Autodesk Inventor part; units mm, degrees
ref_plane "YZ Plane" through (0, 0, 0) normal (1, 0, 0) x (0, 1, 0)
ref_plane "XZ Plane" through (0, 0, 0) normal (0, 1, 0) x (-1, 0, 0)
ref_plane "XY Plane" through (0, 0, 0) normal (0, 0, 1) x (1, 0, 0)
sketch "Sketch1" plane through (0, 0, 0) normal (0, 1, 0) x (-1, 0, 0)
  line L0 (0, 0) -> (-75, 0)
  line L1 (-75, 0) -> (-75, -250)
  line L2 (-75, -250) -> (0, -250)
  line L3 (0, -250) -> (0, 0)
  line L4 (-20, -10) -> (-60, -10)
  line L5 (-60, -10) -> (-60, -15)
  line L6 (-60, -15) -> (-20, -15)
  line L7 (-20, -15) -> (-20, -10)
  line L8 (-75, -125) -> (0, -125) construction
  line L9 (-20, -240) -> (-60, -240)
  line L10 (-60, -240) -> (-60, -235)
  line L11 (-60, -235) -> (-20, -235)
  line L12 (-20, -235) -> (-20, -240)
  line L13 (-75, -35) -> (-265, -35)
  line L14 (-265, -35) -> (-265, -215)
  line L15 (-265, -215) -> (-75, -215)
  line L16 (-75, -215) -> (-75, -35)
  line L17 (-265, -65) -> (-270, -65)
  line L18 (-270, -65) -> (-270, -185)
  line L19 (-270, -185) -> (-265, -185)
  line L20 (-265, -185) -> (-265, -65)
  line L21 (0, -75) -> (-5, -75)
  line L22 (-5, -75) -> (-5, -175)
  line L23 (-5, -175) -> (0, -175)
  line L24 (0, -175) -> (0, -75)
  line L25 (-125, -35) -> (-210, -35)
  line L26 (-210, -35) -> (-210, -15)
  line L27 (-210, -15) -> (-125, -15)
  line L28 (-125, -15) -> (-125, -35)
  line L29 (-125, -215) -> (-210, -215)
  line L30 (-210, -215) -> (-210, -245)
  line L31 (-210, -245) -> (-125, -245)
  line L32 (-125, -245) -> (-125, -215)
  point P0 (-75, -215)
  point P1 (-265, -185)
  point P2 (0, -175)
  dimension "d0" = 75
  dimension "d2" = 40
  dimension "d3" = 5
  dimension "d6" = 190
  dimension "d7" = 180
  dimension "d8" = 5
  dimension "d9" = 120
  dimension "d11" = 20
  dimension "d12" = 5
  dimension "d13" = 100
  dimension "d14" = 75
  dimension "d15" = 85
  dimension "d16" = 50
  dimension "d17" = 10
  dimension "d18" = 30
  dimension "d19" = 230
  dimension "d20" = 35
extrude "Extrusion1" add sketch "Sketch1" along normal blind 5 contours L3 L21 L22 L23 L2 L1 L0 | L1 L15 L14 L13 | L13 L26 L27 L28 | L32 L31 L30 L15 | L14 L19 L18 L17
properties part number "hood"
The model under review builds one solid part; all positions refer to its coordinate system, in mm. Coordinates: 2 decimals unless noted, no trailing zeros. Write each loop counter-clockwise with the first axis right and the second up, starting at its lowest first coordinate (ties: lowest second). Pieces come first, ordered by that corner, then holes. Notation, with made-up numbers: (19, 1.5) - (78, 1.5) arc R24 ccw to (78, 18.5) - close; hole circle Ø8 at (32, 12). An arc over 180 degrees is marked (long way). Answer as a JSON object with one key per item and string values. Group by question number.
1. Add section A-A (x = 50.5). Give the boundary of the cut face in (y, z).
2. Clearance check with flat-ended pins moving along their axes: pin 1 Ø2.5 at (y, z) = (2, -238) entering from +X; pin 2 Ø6 at (x, z) = (220.5, -30.5) entering from -Y. State where each tip first meets the part, or that it passes through.
3. Add section C-C (x = 238.5). Give the boundary of the cut face in (y, z).
4. To check wall thickness, follow probe 1 along Z at (x, y) = (37, 3.7); probe 2 along X at (y, z) = (2.35, -234); probe 3 along X at (y, z) = (2.8, -14). State the ranges of each line that lie inside material, in increasing order.
5. Add section D-D (z = -196.5). Give the boundary of the cut face in (x, y), plus the area to 4 significant figures.
6. Add section B-B (y = 2.5). Give the number of separate pieces and of enclosed holes in the cut face, plus the area to 3 significant figures.
Findings:
{
 "1": {"outline": "(0, -250) - (5, -250) - (5, -240) - (0, -240) - close; (0, -235) - (5, -235) - (5, -15) - (0, -15) - close; (0, -10) - (5, -10) - (5, 0) - (0, 0) - close"},
 "2": {"pin 1": "x = 210", "pin 2": "through"},
 "3": {"outline": "(0, -215) - (5, -215) - (5, -35) - (0, -35) - close"},
 "4": {"probe 1": "-250 to -240, -235 to -15, -10 to 0", "probe 2": "0 to 75, 125 to 210", "probe 3": "0 to 20, 60 to 75"},
 "5": {"outline": "(0, 0) - (265, 0) - (265, 5) - (0, 5) - close", "area": "1,325 mm²"},
 "6": {"separate pieces": "1", "enclosed holes": "2", "area": "56,900 mm²"}
}
